The model under review builds one solid part; all positions refer to its coordinate system, in mm. A direction names the side the tool comes from. Give positions to 0.01 mm unless a question says otherwise; leave off trailing zeros. Order: outer loops, then holes, each group sorted by start corner. A loop starts at its lowest first (then second) coordinate and runs counter-clockwise, first axis right, second up.
Autodesk Inventor part; units mm, degrees
ref_plane "YZ Plane" through (0, 0, 0) normal (1, 0, 0) x (0, 1, 0)
ref_plane "XZ Plane" through (0, 0, 0) normal (0, 1, 0) x (-1, 0, 0)
ref_plane "XY Plane" through (0, 0, 0) normal (0, 0, 1) x (1, 0, 0)
sketch "Sketch1" plane through (0, 0, 0) normal (0, 1, 0) x (-1, 0, 0)
  line L0 (15, -15.715) -> (-15, -15.715)
  line L1 (-15, -15.715) -> (-15, 15.715)
  line L2 (-15, 15.715) -> (15, 15.715)
  line L3 (15, 15.715) -> (15, -15.715)
  point P0 (0, 0)
  dimension "d0" = 30
  dimension "d1" = 31.43
  dimension "d2" = 15
  dimension "d3" = 15.715
extrude "Plate1" add sketch "Sketch1" along normal blind 1.5
sketch "Sketch2" plane through (15, 0, 17.215) normal (0, 0, -1) x (-1, 0, 0)
  line L0 (30, 0) -> (0, 0)
  line L1 (0, 0) -> (0, 45)
  line L2 (0, 45) -> (30, 45)
  line L3 (30, 45) -> (30, 0)
edge flange "Flange1" height 45 angle 90 thickness 1.5 bend radius 0.31 thickness toward (0, 0, -1) relief tear relief width 1.5 relief depth 0.75 edges at (0, 1.5, 15.715) wall of the first edge with corners at (-15, 0, 17.215) (15, 0, 17.215) (15, 45, 17.215) (-15, 45, 17.215)
bend "Bend1"
corner "Corner1"
sketch "Sketch3" plane through (-15, 0, -17.215) normal (0, 0, 1) x (1, 0, 0)
  line L0 (30, 0) -> (0, 0)
  line L1 (0, 0) -> (0, 45)
  line L2 (0, 45) -> (30, 45)
  line L3 (30, 45) -> (30, 0)
edge flange "Flange2" height 45 angle 90 thickness 1.5 bend radius 0.31 thickness toward (0, 0, 1) relief tear relief width 1.5 relief depth 0.75 edges at (0, 1.5, -15.715) wall of the first edge with corners at (15, 0, -17.215) (-15, 0, -17.215) (-15, 45, -17.215) (15, 45, -17.215)
bend "Bend2"
corner "Corner2"
sketch "Sketch6" plane through (-15, 45, 17.215) normal (0, 0, 1) x (1, 0, 0)
  circle A0 centre (15, -10.5) radius 10
  line L0 (5, -10.5) -> (5, 9.5)
  line L1 (5, 9.5) -> (25, 9.5)
  line L2 (25, 9.5) -> (25, -10.5)
  line L3 (0, 0) -> (30, 0)
  line L4 (0, -43.19) -> (0, 0)
  line L5 (5.9376, -6.2723) -> (0, -19)
  line L6 (24.0624, -6.2723) -> (30, -19)
  line L7 (30, -45) -> (0, -45)
  line L8 (30, 0) -> (30, -43.19)
  point P0 (15, -45)
  point P1 (25, 0)
  point P2 (5, -8.2822)
  point P3 (5, 0)
  point P4 (30, -19)
  point P5 (25, -8.2822)
  dimension "d39" = 34.5
  dimension "d40" = 20
  dimension "d41" = 20
  dimension "d42" = 20
  dimension "d43" = 20
  dimension "d45" = 15
  dimension "d48" = 26
  dimension "d49" = 26
  dimension "d50" = 0
extrude "Extrusion1" cut sketch "Sketch6" against normal blind 50 contours A0 L5 L0 L3 L2 L6 | L2 L3 L8 L6 | L5 L4 L3 L0
sketch "Sketch7" plane through (-15, 1.81, 17.215) normal (0, 0, 1) x (1, 0, 0)
  arc A0 (24.0624, 36.9177) -> (5.9376, 36.9177) centre (15, 32.69) ccw
  circle A1 centre (22, 32.69) radius 1.05
  circle A2 centre (15, 39.69) radius 1.05
  circle A3 centre (8, 32.69) radius 1.05
  circle A4 centre (15, 25.69) radius 1.05
  point P0 (15, -1.81)
  dimension "d51" = 7
  dimension "d52" = 2.1
  dimension "d55" = 360
extrude "Extrusion2" cut sketch "Sketch7" against normal blind 20
sketch "Sketch8" plane through (0, 1.5, 0) normal (0, 1, 0) x (1, 0, 0)
  line L0 (15, 15.715) -> (9.0624, 15.715)
  line L1 (9.0624, 15.715) -> (-9.0624, 15.715)
  line L2 (-9.0624, 15.715) -> (-15, 15.715)
  line L3 (-15, 15.715) -> (15, 15.715)
  circle A0 centre (0, -2.285) radius 2.6
  point P0 (0, 0)
  point P1 (7, -2.285)
  point P2 (0, 4.715)
  point P3 (-7, -2.285)
  point P4 (0, -9.285)
  dimension "d59" = 18
  dimension "d60" = 0
  dimension "d61" = 5.2
  dimension "d62" = 7
  dimension "d63" = 0
  dimension "d66" = 360
extrude "Extrusion3" cut sketch "Sketch8" against normal blind 10
sketch "Sketch9" plane through (0, 1.5, 0) normal (0, 1, 0) x (1, 0, 0)
  point P0 (0, 0)
hole "Hole3" at (0, 1.5, -4.715) at (7, 1.5, 2.285) at (-7, 1.5, 2.285) at (0, 1.5, 9.285) direction (0, -1, 0) diameter 2.1 depth 1.5
hole "Hole4" at (0, 34.5, 17.215) direction (0, 0, -1) diameter 5.2 depth 1.5
sketch "Sketch10" plane through (15, 1.81, -17.215) normal (0, 0, -1) x (-1, 0, 0)
  circle A0 centre (15, 32.69) radius 2.6
  point P0 (15, -1.81)
hole "Hole5" at (0, 34.5, -17.215) direction (0, 0, 1) diameter 5 depth 1.5
equation "\"d75\" = Thickness"
equation "\"d82\" = Thickness"
equation "\"d89\" = Thickness"
equation "\"d4\" = Thickness"
equation "\"d5\" = BendReliefWidth"
equation "\"d6\" = BendReliefDepth"
equation "\"d7\" = MinimumRemnant"
equation "\"d8\" = TransitionRadius"
equation "\"d11\" = BendRadius"
equation "\"d12\" = CornerReliefSize"
equation "\"d13\" = GapSize"
equation "\"d14\" = JacobiRadiusSize"
equation "\"d15\" = BendReliefWidth"
equation "\"d16\" = BendReliefDepth"
equation "\"d17\" = MinimumRemnant"
equation "\"d18\" = TransitionRadius"
equation "\"d21\" = BendRadius"
equation "\"d22\" = CornerReliefSize"
equation "\"d23\" = GapSize"
equation "\"d24\" = JacobiRadiusSize"
equation "\"BendReliefWidth\" = Thickness"
equation "\"BendReliefDepth\" = 0.5 * Thickness"
equation "\"CornerReliefSize\" = 4 * Thickness"
equation "\"MinimumRemnant\" = 2 * Thickness"
equation "\"TransitionRadius\" = BendRadius"
equation "\"JacobiRadiusSize\" = BendRadius"
equation "\"GapSize\" = Thickness"
properties part number "axis_7_top_frame" material "Aluminum 6061-AHC"
1. Take a section at A-A (y = 15). Write out the cut boundary in (x, z) (3 decimals), and give its area (3 significant figures).
2. Take a section at D-D (z = -7). Write out the cut boundary in (x, y), and give its area (3 significant figures).
3. Take a section at B-B (x = -7). Write out the cut boundary in (y, z) (3 decimals), and give its area (3 significant figures).
4. To check wall thickness, follow line 1 (Z direction, x = -8, y = 10.5) (3 decimals); line 2 (Z direction, x = 0, y = 0.75) (3 decimals); line 3 (Y direction, x = 2.5, z = -1.5). State the ranges of each line that lie inside material, in increasing order.
5. For faces 5 (the flat face through (0, 23, -15.715)), 6 (the flat face through (-15, 1, 0)), list the 3-axis set-ups (+Z, -Z, +X, -X, +Y, -Y) from which the entire face can be reached by the end or side of a thin tool; tool diameter is ignored.
6. Insertion check: pin 1 (6 mm diameter, centred on x = 0, y = 34.5, fed in from +Z) (3 decimals); pin 2 (2.5 mm diameter, centred on x = -7, z = 2.285, fed in from +Y); pin 3 (1.3 mm diameter, centred on x = -7, y = 34.5, fed in from +Z) (3 decimals). Each pin has a flat end and moves straight along its axis. Give the tip position at first contact, or say it passes through.
7. Draft analysis for pull direction Y (two halves, no side actions). For faces 1 (the flat face through (11.99, 32.45, -16.45)), 2 (the cylindrical face through (6.772, 33.475, 16.476)), 3 (the cylindrical face through (-0.1, 37.1, 16.5)), 4 (the flat face through (0, 19, 17.215)), state which applies: pulls with the +Y half, pulls with the -Y half, needs draft (parallel to the pull), parting line crosses it, or undercut.
8. Take a section at C-C (y = 27.5). Write out the cut boundary in (x, z) (3 decimals).
Answer:
1. outline: (-15, -17.215) - (15, -17.215) - (15, -15.715) - (-15, -15.715) - close; (-15, 15.715) - (15, 15.715) - (15, 17.215) - (-15, 17.215) - close
1. area: 90.0 mm2
2. outline: (-15, 0) - (15, 0) - (15, 1.5) - (-15, 1.5) - close
2. area: 45.0 mm2
3. outline: (0, -15.405) arc R1.81 ccw to (1.81, -17.215) - (41.641, -17.215) - (41.641, -15.715) - (1.81, -15.715) arc R0.31 cw to (1.5, -15.405) - (1.5, 1.235) - (0, 1.235) - close; (0, 3.335) - (1.5, 3.335) - (1.5, 15.405) arc R0.31 cw to (1.81, 15.715) - (33.45, 15.715) - (33.45, 17.215) - (1.81, 17.215) arc R1.81 ccw to (0, 15.405) - close; (35.55, 15.715) - (41.641, 15.715) - (41.641, 17.215) - (35.55, 17.215) - close
3. area: 164 mm2
4. line 1: z = -17.215 to -15.715, 15.715 to 17.215
4. line 2: z = -16.872 to -5.765, -3.665 to -0.315, 4.885 to 8.235, 10.335 to 16.872
4. line 3: y = 0 to 1.5
5. face 5: +X, -X, +Y
5. face 6: +Z, -Z, -X, +Y, -Y
6. pin 1: stops at z = 17.215
6. pin 2: stops at y = 1.5
6. pin 3: stops at z = -15.715
7. face 1: pulls with the +Y half
7. face 2: undercut
7. face 3: undercut
7. face 4: needs draft
8. outline: (-14.3, -17.215) - (14.3, -17.215) - (14.3, -15.715) - (-14.3, -15.715) - close; (-14.3, 15.715) - (-1.05, 15.715) - (-1.05, 17.215) - (-14.3, 17.215) - close; (1.05, 15.715) - (14.3, 15.715) - (14.3, 17.215) - (1.05, 17.215) - close
